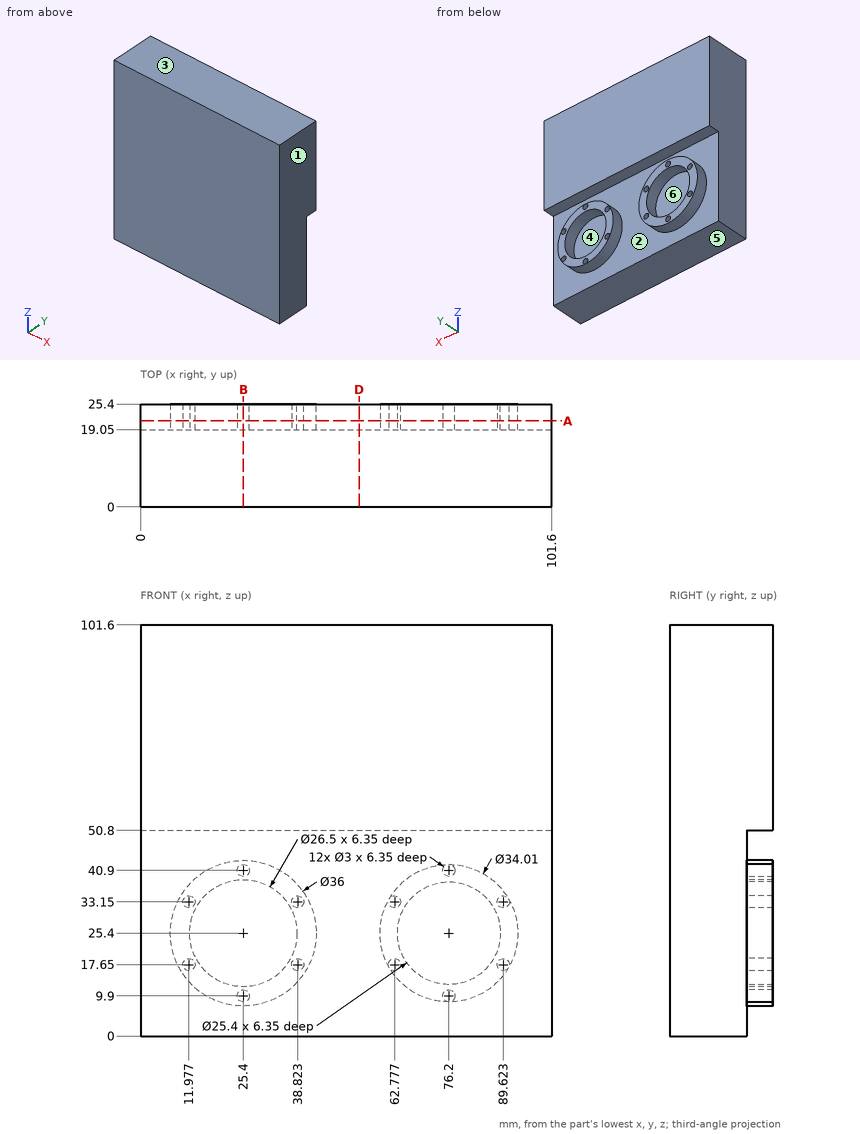
Source: three-view drawing plus pictorial views. Frame: mm from the lowest corner of the part. A direction names the side the tool comes from. Coordinates: 2 decimals unless noted, no trailing zeros. Loops run counter-clockwise (first coordinate to the right, second up) from the corner with the lowest first, then second, coordinate; pieces in that order, holes last. Notation, with made-up numbers: (75, -4) -> (109, -4) arc R31 cw to (109, 24) -> close; hole circle Ø7 at (2, 69.5). An arc over 180 degrees is marked (long way). Answer in a Markdown table with one row per item. Add a question column.
Q1. Pull-direction query (X, two-part tool) for the marked faces 1, 2, 3 and 4; classes: pulls with the +X half, pulls with the -X half, needs draft (parallel to the pull), parting line crosses it, or undercut.
Q2. Section B-B on x = 25.4. Return the cut outline in (y, z), and give its area (3 significant figures).
Q3. Ray query, line 1 along Z through (x, y) = (22, 19.5) (1 decimal); line 2 along Y through (x, z) = (43.5, 9); line 3 along Z through (x, y) = (68, 23.5). Return the intervals inside material, ascending.
Q4. Section A-A on y = 21.25. Give the number of separate pieces and of enclosed holes in the cut face.
Q5. Contact query for a flat-ended pin moving along its axis: pin 1 Ø12.5 at (x, z) = (71, 26) entering from +Y. Output: stop coordinate, or through.
Q6. Section D-D on x = 54. Return the cut outline in (y, z), and give its area (3 significant figures).
Q7. Reachability of the marked faces 5 and 6 from +Z, -Z, +X, -X, +Y, -Y: full face, straight path, thin tool, end or side. Return the list, or none.
Computed values:
| question | item | result |
|---|---|---|
| 1 | face 1 | pulls with the +X half |
| 1 | face 2 | undercut |
| 1 | face 3 | needs draft |
| 1 | face 4 | undercut |
| 2 | outline | (0, 0) -> (19.05, 0) -> (19.05, 7.4) -> (25.4, 7.4) -> (25.4, 8.4) -> (19.05, 8.4) -> (19.05, 11.4) -> (25.4, 11.4) -> (25.4, 12.15) -> (19.05, 12.15) -> (19.05, 38.65) -> (25.4, 38.65) -> (25.4, 39.4) -> (19.05, 39.4) -> (19.05, 42.4) -> (25.4, 42.4) -> (25.4, 43.4) -> (19.05, 43.4) -> (19.05, 50.8) -> (25.4, 50.8) -> (25.4, 101.6) -> (0, 101.6) -> close |
| 2 | area | 2,280 mm^2 |
| 3 | line 1 | z = 7.7 to 12.6, 38.2 to 43.1, 50.8 to 101.6 |
| 3 | line 2 | y = 0 to 19.05 |
| 3 | line 3 | z = 10.5 to 15.7, 35.1 to 40.3, 50.8 to 101.6 |
| 4 | separate pieces | 3 |
| 4 | enclosed holes | 14 |
| 5 | pin 1 | stops at y = 19.05 |
| 6 | outline | (0, 0) -> (19.05, 0) -> (19.05, 50.8) -> (25.4, 50.8) -> (25.4, 101.6) -> (0, 101.6) -> close |
| 6 | area | 2,260 mm^2 |
| 7 | face 5 | -Z, +X, -X, +Y, -Y |
| 7 | face 6 | +Y |
